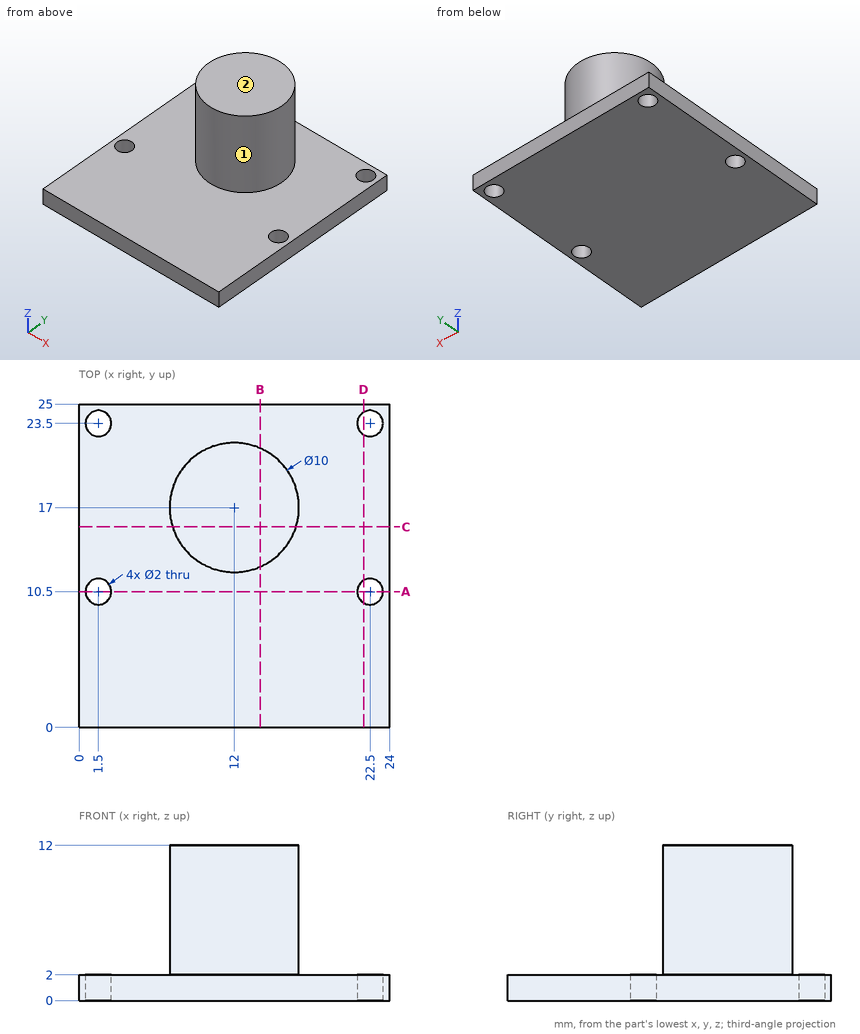
Study the drawing (mm; zero at the part's minimum x, y, z) and answer. A direction names the side the tool comes from. Give positions to 0.01 mm unless a question says otherwise; leave off trailing zeros. Write each loop counter-clockwise with the first axis right and the second up, starting at its lowest first coordinate (ties: lowest second). Pieces come first, ordered by that corner, then holes. Notation, with made-up numbers: (10.25, 44.25) - (35.25, 44.25) arc R11 ccw to (35.25, 54.25) - close; hole circle Ø5 at (86.25, 77). An arc over 180 degrees is marked (long way). One line per question, with ' | ' between items. Start each with the question number.
1. Given P1, Ø5, axis at x = 9.5, y = 12, coming from the -Z side; P2, Ø5, axis at x = 8.5, z = 5.5, coming from the +Y side; P3, Ø1.8, axis at x = 22.5, y = 23.5, coming from the -Z side; P4, Ø2, axis at y = 16.5, z = 9, coming from the +X side, each flat-ended and moving along its own axis, determine where each tip first touches the part or whether it passes through.
2. Section D-D, the plane x = 22 is taken. Determine the outline of the cut face in (y, z), then the cut area to 3 significant figures.
3. Section C-C, the plane y = 15.5 is taken. Determine the outline of the cut face in (x, z), then the cut area to 3 significant figures.
4. Section A-A, the plane y = 10.5 is taken. Determine the outline of the cut face in (x, z), then the cut area to 3 significant figures.
5. Section B-B, the plane x = 14 is taken. Determine the outline of the cut face in (y, z).
6. Straight lines are drawn through the part: line 1 (Y direction, x = 1.5, z = 0.8); line 2 (Z direction, x = 4.5, y = 22.5); line 3 (Y direction, x = 8.25, z = 2.5). For each, find the intervals that lie inside material, in ascending order.
7. For the marked faces 1 and 2, determine the directions among +Z, -Z, +X, -X, +Y, -Y from which every point of the face is accessible in a straight line to the end or side of a thin tool.
Result:
1) P1: stops at z = 0 | P2: stops at y = 21.9 | P3: passes through | P4: stops at x = 17
2) outline: (0, 0) - (9.63, 0) - (9.63, 2) - (0, 2) - close; (11.37, 0) - (22.63, 0) - (22.63, 2) - (11.37, 2) - close; (24.37, 0) - (25, 0) - (25, 2) - (24.37, 2) - close | area: 43.1 mm2
3) outline: (0, 0) - (24, 0) - (24, 2) - (16.77, 2) - (16.77, 12) - (7.23, 12) - (7.23, 2) - (0, 2) - close | area: 143 mm2
4) outline: (0, 0) - (0.5, 0) - (0.5, 2) - (0, 2) - close; (2.5, 0) - (21.5, 0) - (21.5, 2) - (2.5, 2) - close; (23.5, 0) - (24, 0) - (24, 2) - (23.5, 2) - close | area: 40.0 mm2
5) outline: (0, 0) - (25, 0) - (25, 2) - (21.58, 2) - (21.58, 12) - (12.42, 12) - (12.42, 2) - (0, 2) - close
6) line 1: y = 0 to 9.5, 11.5 to 22.5, 24.5 to 25 | line 2: z = 0 to 2 | line 3: y = 13.69 to 20.31
7) face 1: +Z | face 2: +Z, +X, -X, +Y, -Y
